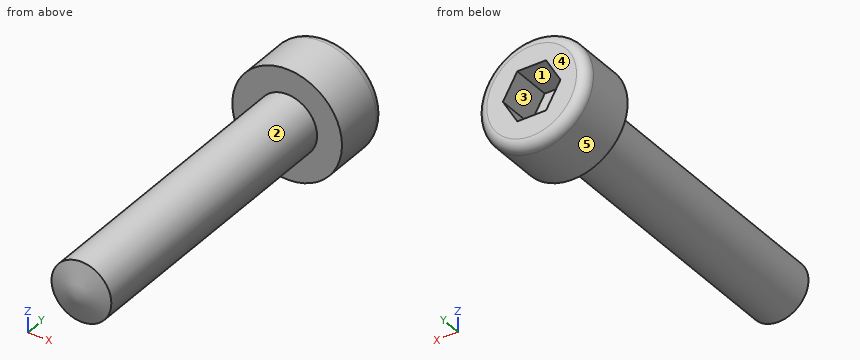
```python
from build123d import *

# Parameters (mm, degrees)
CUT_EXTRUDE1_DEPTH = 2


with BuildPart() as part:
    # Sketch1 → Base-Revolve (revolve)
    with BuildSketch(Plane.XY):
        with BuildLine():
            Line((0, -15.401923789), (0, 3))
            Line((0, 3), (2.25, 3))
            ThreePointArc((2.25, 3), (2.603553391, 2.853553391), (2.75, 2.5))
            Line((2.75, 2.5), (2.75, 0))
            Line((2.75, 0), (1.5, 0))
            Line((1.5, 0), (1.5, -15))
            Line((1.5, -15), (0, -15.401923789))
        make_face()
    revolve(axis=Axis((0, 3, 0), (0, 1, 0)))

    # Sketch2 → Cut-Extrude1 (cut)
    with BuildSketch(Plane(origin=(0, 3, 0), x_dir=(-1, 0, 0), z_dir=(0, 1, 0))):
        Polygon((-1.443375673, 0), (-0.721687836, -1.25), (0.721687836, -1.25), (1.443375673, 0), (0.721687836, 1.25), (-0.721687836, 1.25), align=None)
    extrude(amount=-CUT_EXTRUDE1_DEPTH, mode=Mode.SUBTRACT)


solid = part.part
```
CAD build for the part. Positions are in the model's coordinates, mm. Face numbers are marked on the shaded views. A direction names the side the tool comes from. Round coordinates to 2 decimals unless told otherwise and drop trailing zeros. Write each loop counter-clockwise with the first axis right and the second up, starting at its lowest first coordinate (ties: lowest second). Pieces come first, ordered by that corner, then holes. Notation, with made-up numbers: (27, -35.75) - (55, -35.75) arc R11 ccw to (55, -30.75) - close; hole circle Ø1 at (84.25, 69). An arc over 180 degrees is marked (long way). Return JSON: item names as keys, results as strings. Group by question number.
Item 1: 3-axis set-ups, long thin cutter, end or side, ignore diameter. For the marked faces 1 and 2: which of +Z, -Z, +X, -X, +Y, -Y reach the whole face in a straight line?
Item 2: Probe probe 1 along Z at (x, y) = (-0.1, 2); probe 2 along Y at (x, z) = (-1.55, 0.25); probe 3 along X at (y, z) = (-1.5, 0.55). List the from-to ranges inside material, lowest first.
Item 3: Band-saw the part on A-A on y = -6.5. List the corners of the cut face in (x, z).
Item 4: Mould opens along X. For the marked faces 3, 4 and 5 say: +X half, -X half, draft (parallel to the pull), parting line (faces both ways), or undercut.
Item 5: Flat gauge pins, fed straight in: pin 1 Ø2 at (x, z) = (0.5, 0.5) entering from +Y; pin 2 Ø1 at (y, z) = (-7, 1.5) entering from -X; pin 3 Ø1.5 at (x, z) = (1.5, -1.5) entering from -Y; pin 4 Ø1 at (x, z) = (-0.5, 1) entering from -Y. Where does each tip first touch, or does it go through?
Resolved:
{
 "1": {"face 1": "+Y", "face 2": "-Y"},
 "2": {"probe 1": "z = -2.75 to -1.25, 1.25 to 2.75", "probe 2": "y = 0 to 3", "probe 3": "x = -1.4 to 1.4"},
 "3": {"outline": "circle Ø3 at (0, 0)"},
 "4": {"face 3": "undercut", "face 4": "draft", "face 5": "parting line"},
 "5": {"pin 1": "stops at y = 3", "pin 2": "stops at x = -1.12", "pin 3": "stops at y = -15.03", "pin 4": "stops at y = -15.24"}
}
